Answer from the drawing. Dimensions are ordinates in mm from the lowest x, y and z of the part. Give positions to 0.01 mm unless a question says otherwise; leave off trailing zeros. Order: outer loops, then holes, each group sorted by start corner. A loop starts at its lowest first (then second) coordinate and runs counter-clockwise, first axis right, second up.
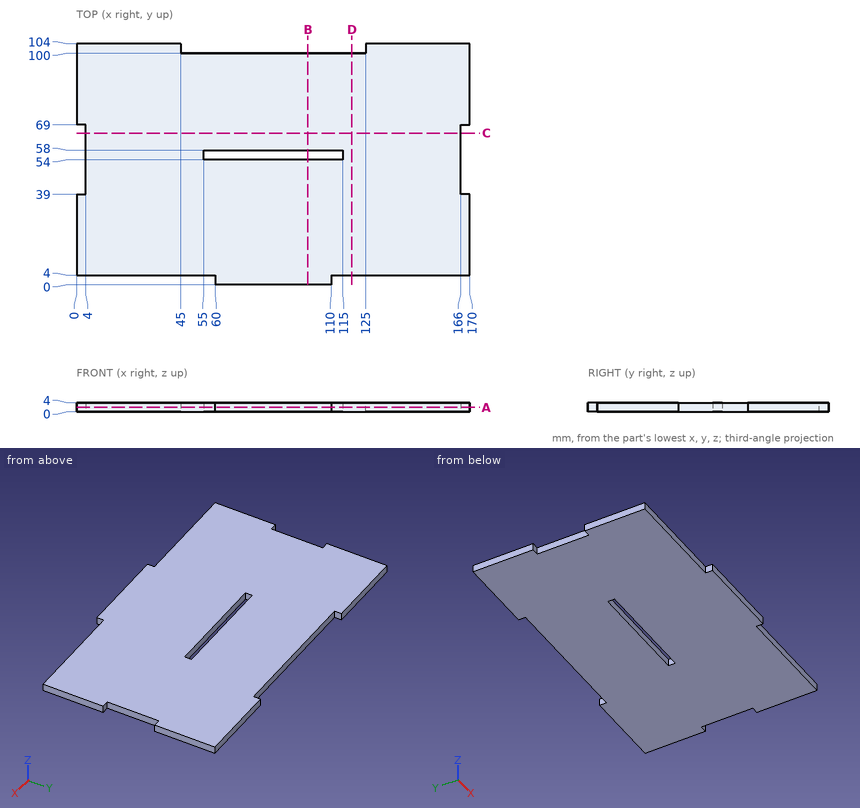
1. Straight lines are drawn through the part: probe 1 along Y at (x, z) = (104, 0.45); probe 2 along Y at (x, z) = (56, 2.75); probe 3 along Y at (x, z) = (54, 2.3). For each, find the intervals that lie inside material, in ascending order.
Findings below:
probe 1: y = 0 to 54, 58 to 100
probe 2: y = 4 to 54, 58 to 100
probe 3: y = 4 to 100
2. The part is cut by section A-A (z = 1.95). Write down the section's boundary in (x, y), then the cut area to 3 significant figures.
Findings below:
outline: (0, 4) - (60, 4) - (60, 0) - (110, 0) - (110, 4) - (170, 4) - (170, 39) - (166, 39) - (166, 69) - (170, 69) - (170, 104) - (125, 104) - (125, 100) - (45, 100) - (45, 104) - (0, 104) - (0, 69) - (4, 69) - (4, 39) - (0, 39) - close; hole (55, 54) - (115, 54) - (115, 58) - (55, 58) - close
area: 16,400 mm2
3. The part is cut by section C-C (y = 65.5). Write down the section's boundary in (x, z).
Findings below:
outline: (4, 0) - (166, 0) - (166, 4) - (4, 4) - close
4. The part is cut by section D-D (x = 119). Write down the section's boundary in (y, z).
Findings below:
outline: (4, 0) - (100, 0) - (100, 4) - (4, 4) - close
5. The part is cut by section B-B (x = 100). Write down the section's boundary in (y, z), then the cut area to 3 significant figures.
Findings below:
outline: (0, 0) - (54, 0) - (54, 4) - (0, 4) - close; (58, 0) - (100, 0) - (100, 4) - (58, 4) - close
area: 384 mm2
6. Given P1, Ø1.2, axis at y = 102, z = 2, coming from the -X side; P2, Ø1.2, axis at x = 90, z = 2.5, coming from the +Y side; P3, Ø2, axis at y = 55.5, z = 2, coming from the +X side; P4, Ø1.2, axis at y = 48, z = 1.5, coming from the -X side, each flat-ended and moving along its own axis, determine where each tip first touches the part or whether it passes through.
Findings below:
P1: stops at x = 0
P2: stops at y = 100
P3: stops at x = 166
P4: stops at x = 4
